The drawing under review shows one solid part. Ordinate dimensions are in mm from its lowest x, y, z. Coordinates: 2 decimals unless noted, no trailing zeros. Order: outer loops, then holes, each group sorted by start corner. A loop starts at its lowest first (then second) coordinate and runs counter-clockwise, first axis right, second up.
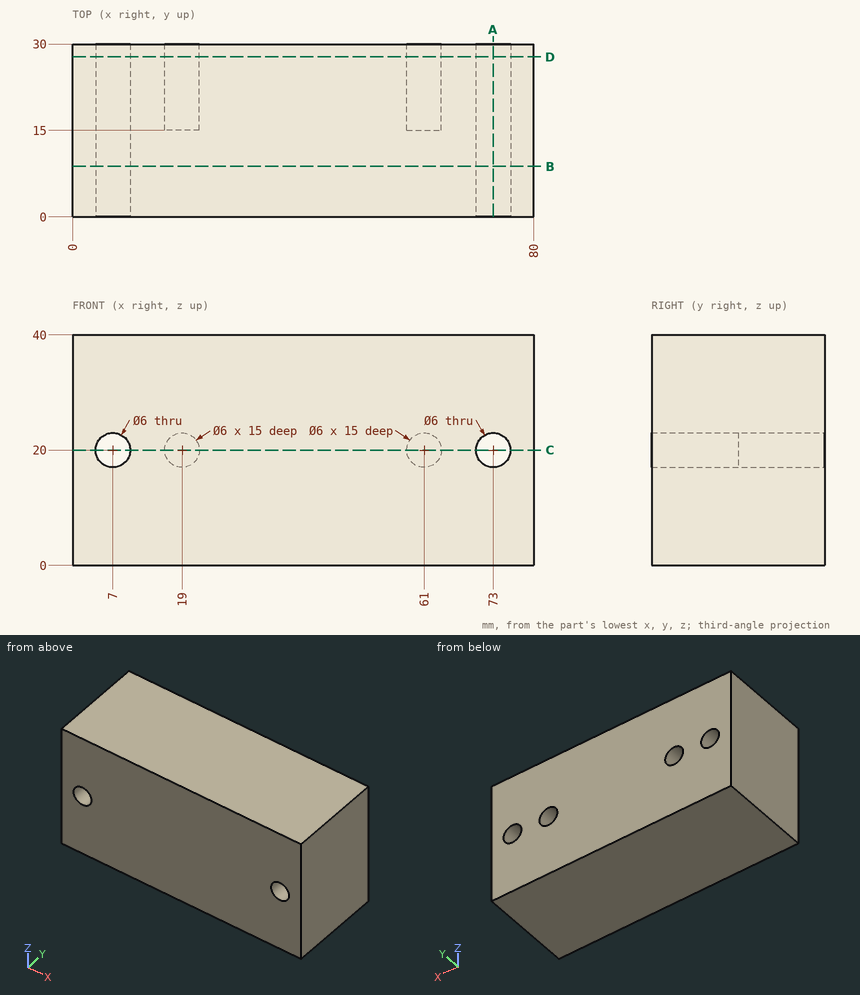
(1) Wall thickness on probe 1 along X at (y, z) = (19, 20); probe 2 along Z at (x, y) = (61, 19.75); probe 3 along Z at (x, y) = (75, 3.25): over which ranges is each line inside the solid? List them lowest first.
A:
probe 1: x = 0 to 4, 10 to 16, 22 to 58, 64 to 70, 76 to 80
probe 2: z = 0 to 17, 23 to 40
probe 3: z = 0 to 17.76, 22.24 to 40
(2) We need section D-D, the plane y = 27.75. Write out the cut boundary in (x, z).
A:
outline: (0, 0) - (80, 0) - (80, 40) - (0, 40) - close; hole circle Ø6 at (7, 20); hole circle Ø6 at (19, 20); hole circle Ø6 at (61, 20); hole circle Ø6 at (73, 20)
(3) We need section B-B, the plane y = 8.75. Write out the cut boundary in (x, z), and give its area (3 significant figures).
A:
outline: (0, 0) - (80, 0) - (80, 40) - (0, 40) - close; hole circle Ø6 at (7, 20); hole circle Ø6 at (73, 20)
area: 3,140 mm2
(4) We need section C-C, the plane z = 20. Write out the cut boundary in (x, y).
A:
outline: (0, 0) - (4, 0) - (4, 30) - (0, 30) - close; (10, 0) - (70, 0) - (70, 30) - (64, 30) - (64, 15) - (58, 15) - (58, 30) - (22, 30) - (22, 15) - (16, 15) - (16, 30) - (10, 30) - close; (76, 0) - (80, 0) - (80, 30) - (76, 30) - close
(5) For pin 1 Ø1.5 at (x, y) = (13.5, 26.5) entering from -Z; pin 2 Ø3.5 at (x, z) = (61, 20) entering from +Y, all flat-tipped, find the tip position at first contact; note any pin that passes through.
A:
pin 1: stops at z = 0
pin 2: stops at y = 15
(6) We need section A-A, the plane x = 73. Write out the cut boundary in (y, z).
A:
outline: (0, 0) - (30, 0) - (30, 17) - (0, 17) - close; (0, 23) - (30, 23) - (30, 40) - (0, 40) - close
